The listing builds one solid part. Answer for the finished solid, in the listing's coordinates (mm). Round coordinates to 2 decimals unless told otherwise and drop trailing zeros. Loops run counter-clockwise (first coordinate to the right, second up) from the corner with the lowest first, then second, coordinate; pieces in that order, holes last. Notation, with made-up numbers: (67.25, 24) -> (81.25, 24) arc R15 ccw to (81.25, 39) -> close; hole circle Ø5 at (61, 13.25). An arc over 180 degrees is marked (long way). Write each question's results on one line, items separated by ' | '. Start each with the question number.
(1) The part is cut by section B-B (x = -55). Determine the outline of the cut face in (y, z), plus the area to 3 significant figures.
(2) The part is cut by section D-D (y = -42). Determine the outline of the cut face in (x, z), plus the area to 3 significant figures.
(3) The part is cut by section A-A (z = 0.7). Determine the outline of the cut face in (x, y), plus the area to 3 significant figures.
(4) Straight lines are drawn through the part: probe 1 along X at (y, z) = (-39.5, 0.4); probe 2 along Y at (x, z) = (-55, 0.1); probe 3 along Y at (x, z) = (-28.5, 0.45). For each, find the intervals that lie inside material, in ascending order.
(5) The part is cut by section C-C (y = -48). Determine the outline of the cut face in (x, z), plus the area to 3 significant figures.
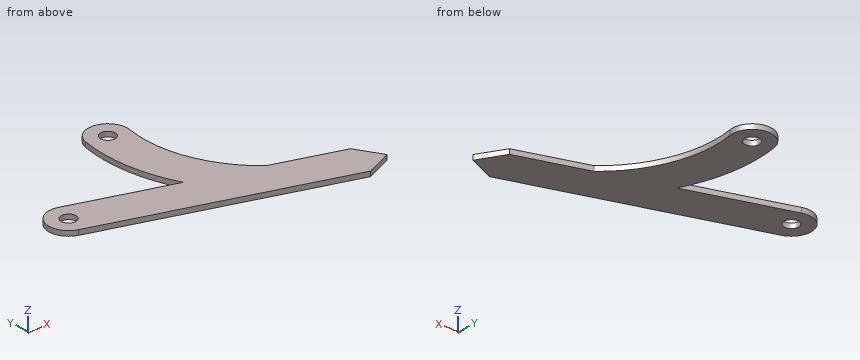
```python
from build123d import *

# Parameters (mm, degrees)
ESQUISSE1_R               = 1.5
T_LE_DE_BASE_PLI_E1_DEPTH = 1


# Sheet-metal steps are written as plain solids
with BuildPart() as part:
    # Esquisse1 → Tôle de base pliée1 (new body)
    with BuildSketch(Plane.XY):
        with BuildLine():
            Line((-53.194732382, -46.443882138), (-33.149125492, -53.169374239))
            ThreePointArc((-33.149125492, -53.169374239), (-36.034099594, -43.334809734), (-35.67163719, -33.092234102))
            ThreePointArc((-35.67163719, -33.092234102), (-30.970075892, -29.94655113), (-27.82439292, -34.648112428))
            ThreePointArc((-27.82439292, -34.648112428), (-26.960351912, -47.211264855), (-19.876250068, -57.622550405))
            Line((-19.876250068, -57.622550405), (-6.239220274, -62.197903832))
            Line((-6.239220274, -62.197903832), (-3.271691792, -67.412668899))
            Line((-3.271691792, -67.412668899), (-8.783892369, -69.782404075))
            Line((-8.783892369, -69.782404075), (-55.739404477, -54.02838238))
            ThreePointArc((-55.739404477, -54.02838238), (-58.259318551, -48.963796212), (-53.194732382, -46.443882138))
        make_face()
        with Locations((-54.467068429, -50.236132259)):
            Circle(ESQUISSE1_R, mode=Mode.SUBTRACT)
        with Locations((-31.748015055, -33.870173265)):
            Circle(ESQUISSE1_R, mode=Mode.SUBTRACT)
    extrude(amount=T_LE_DE_BASE_PLI_E1_DEPTH)


solid = part.part
```
Checked values:
1) outline: (-54.28, 0) -> (-51.64, 0) -> (-51.64, 1) -> (-54.28, 1) -> close; (-48.83, 0) -> (-46.27, 0) -> (-46.27, 1) -> (-48.83, 1) -> close | area: 5.20 mm2
2) outline: (-36.17, 0) -> (-28.14, 0) -> (-28.14, 1) -> (-36.17, 1) -> close | area: 8.04 mm2
3) outline: (-55.74, -54.03) -> (-8.78, -69.78) -> (-3.27, -67.41) -> (-6.24, -62.2) -> (-19.88, -57.62) arc R24.09 cw to (-27.82, -34.65) arc R4 ccw to (-35.67, -33.09) arc R32.09 ccw to (-33.15, -53.17) -> (-53.19, -46.44) arc R4 ccw to start; hole circle Ø3 at (-54.47, -50.24); hole circle Ø3 at (-31.75, -33.87) | area: 630 mm2
4) probe 1: x = -36.28 to -28.28 | probe 2: y = -54.28 to -51.64, -48.83 to -46.27 | probe 3: y = -63.17 to -31.54
5) outline: (-57.78, 0) -> (-48.56, 0) -> (-48.56, 1) -> (-57.78, 1) -> close; (-35.09, 0) -> (-26.67, 0) -> (-26.67, 1) -> (-35.09, 1) -> close | area: 17.6 mm2
